Design review of the part shown in the three views and the two pictorial views. Dimensions are in mm from the part's minimum x, y and z. A direction names the side the tool comes from. Coordinates: 2 decimals unless noted, no trailing zeros. Write each loop counter-clockwise with the first axis right and the second up, starting at its lowest first coordinate (ties: lowest second). Pieces come first, ordered by that corner, then holes. Notation, with made-up numbers: (39.5, -22.5) -> (70.5, -22.5) arc R13 ccw to (70.5, -3.5) -> close; hole circle Ø1 at (-23, -40). An arc over 180 degrees is marked (long way). Write item = value, one per line. Start each with the question number.
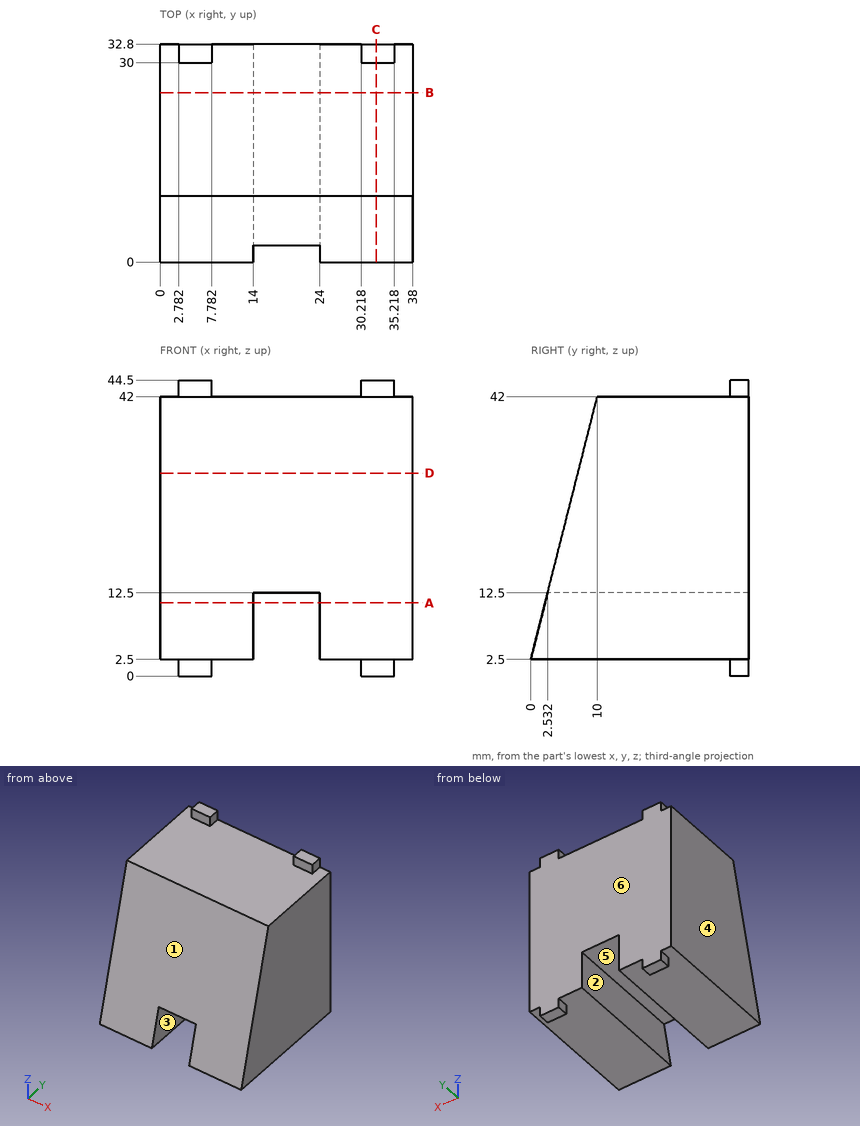
(1) For pin 1 Ø0.8 at (y, z) = (31, 0.5) entering from +X; pin 2 Ø1.2 at (y, z) = (31.5, 1) entering from -X; pin 3 Ø12 at (x, z) = (4.5, 31.5) entering from -Y, all flat-tipped, find the tip position at first contact; note any pin that passes through.
(2) For the marked faces 5 and 6, list the 3-axis set-ups (+Z, -Z, +X, -X, +Y, -Y) from which the entire face can be reached by the end or side of a thin tool; tool diameter is ignored.
(3) Take a section at C-C, the plane x = 32.5. State the section outline as (y, z) points, then the cut area to 3 significant figures.
(4) Mouldability with a two-part tool opening along X and no side actions: class the marked faces 1, 2, 3 and 4 as pulls with the +X half, pulls with the -X half, needs draft (parallel to the pull), parting line crosses it, or undercut.
(5) Take a section at A-A, the plane z = 11. State the section outline as (x, y) points.
(6) Take a section at D-D, the plane z = 30.5. State the section outline as (x, y) points, then the cut area to 3 significant figures.
(7) Take a section at B-B, the plane y = 25.5. State the section outline as (x, z) points, then the cut area to 3 significant figures.
(8) For line 1 (X direction, y = 6, z = 5); line 2 (Z direction, x = 30, y = 17); line 3 (Z direction, x = 16, y = 31.5), list the stretches that pass through material, from the lowest coordinate up.
Report:
q1.pin_1 = 35.22
q1.pin_2 = 2.78
q1.pin_3 = 5.82
q2.face_5 = -Z, +Y, -Y
q2.face_6 = +Z, -Z, +X, -X, +Y
q3.outline = (0, 2.5) -> (30, 2.5) -> (30, 0) -> (32.8, 0) -> (32.8, 44.5) -> (30, 44.5) -> (30, 42) -> (10, 42) -> close
q3.area = 1,110 mm2
q4.face_1 = needs draft
q4.face_2 = undercut
q4.face_3 = undercut
q4.face_4 = pulls with the -X half
q5.outline = (0, 2.15) -> (14, 2.15) -> (14, 32.8) -> (0, 32.8) -> close; (24, 2.15) -> (38, 2.15) -> (38, 32.8) -> (24, 32.8) -> close
q6.outline = (0, 7.09) -> (38, 7.09) -> (38, 32.8) -> (0, 32.8) -> close
q6.area = 977 mm2
q7.outline = (0, 2.5) -> (14, 2.5) -> (14, 12.5) -> (24, 12.5) -> (24, 2.5) -> (38, 2.5) -> (38, 42) -> (0, 42) -> close
q7.area = 1,400 mm2
q8.line_1 = 0 to 14, 24 to 38
q8.line_2 = 2.5 to 42
q8.line_3 = 12.5 to 42
